The listing builds one solid part. Answer for the finished solid, in the listing's coordinates (mm). A direction names the side the tool comes from. Give positions to 0.01 mm unless a question says otherwise; leave off trailing zeros. Write each loop counter-clockwise with the first axis right and the second up, starting at its lowest first coordinate (ties: lowest second). Pieces come first, ordered by that corner, then holes.
```python
from build123d import *

# Parameters (mm, degrees)
BOSS_EXTRUDE1_DEPTH = 1.524


with BuildPart() as part:
    # Sketch1 → Boss-Extrude1 (new body)
    with BuildSketch(Plane.XY):
        with BuildLine():
            Line((82.44470135, -1.524), (82.44470135, 0))
            Line((82.44470135, 0), (51.403450054, 0))
            ThreePointArc((51.403450054, 0), (63.788927887, 14.019916875), (82.44470135, 12.634187153))
            ThreePointArc((82.44470135, 12.634187153), (98.093428139, 9.137765846), (111.269499156, 0))
            Line((111.269499156, 0), (111.269499156, -1.524))
            ThreePointArc((111.269499156, -1.524), (98.093428139, -10.661765846), (82.44470135, -14.158187153))
            ThreePointArc((82.44470135, -14.158187153), (63.788927887, -15.543916875), (51.403450054, -1.524))
            Line((51.403450054, -1.524), (82.44470135, -1.524))
        make_face()
    extrude(amount=BOSS_EXTRUDE1_DEPTH)


solid = part.part
```
Item 1: A cutting plane is placed at A-A, the plane x = 68. Give the vertices of the cut face in (y, z).
Conclusion:
outline: (-16.76, 0) - (-1.52, 0) - (-1.52, 1.52) - (-16.76, 1.52) - close; (0, 0) - (15.24, 0) - (15.24, 1.52) - (0, 1.52) - close
Item 2: Determine the mould class of faces 3 (the face through (97.886, 9.228, 0.751)), 4 (the face through (82, -4, 1.524)), 5 (the face through (67, -1.524, 1)) for opening direction Y: pulls with the +Y half, pulls with the -Y half, needs draft (parallel to the pull), parting line crosses it, or undercut.
Conclusion:
face 3: pulls with the +Y half
face 4: needs draft
face 5: undercut
Item 3: A cutting plane is placed at C-C, the plane x = 61.5. Give the vertices of the cut face in (y, z), plus the area to 3 significant figures.
Conclusion:
outline: (-14.45, 0) - (-1.52, 0) - (-1.52, 1.52) - (-14.45, 1.52) - close; (0, 0) - (12.92, 0) - (12.92, 1.52) - (0, 1.52) - close
area: 39.4 mm2
Item 4: Consider probe 1 along Y at (x, z) = (80, 1.25); probe 2 along Y at (x, z) = (73, 0.55); probe 3 along X at (y, z) = (2, 0.9). Determine where each line is inside the solid, lowest interval first.
Conclusion:
probe 1: y = -15.4 to -1.52, 0 to 13.87
probe 2: y = -17.06 to -1.52, 0 to 15.53
probe 3: x = 52.05 to 109.19
Item 5: A cutting plane is placed at B-B, the plane z = 1.05. Give the vertices of the cut face in (x, y), plus the area to 3 significant figures.
Conclusion:
outline: (51.4, -1.52) arc R21.04 ccw to (82.44, -14.16) arc R41.74 ccw to (111.27, -1.52) - (111.27, 0) arc R41.74 ccw to (82.44, 12.63) arc R21.04 ccw to (51.4, 0) - (82.44, 0) - (82.44, -1.52) - close
area: 1,320 mm2
Item 6: Which of the six approach directions +Z, -Z, +X, -X, +Y, -Y give full straight-line access (tool end or side, diameter ignored) to faces 1 (the face through (82, -4, 0)), 2 (the face through (67, 0, 1))?
Conclusion:
face 1: -Z, +X, -X, +Y, -Y
face 2: +Z, -Z, -X
Item 7: Each of these flat-tipped pins is pushed along its axis until it touches: P1, Ø0.8, axis at x = 67.5, z = 1, coming from the +Y side; P2, Ø0.5, axis at x = 61, z = 0.5, coming from the -Y side; P3, Ø0.8, axis at y = -0.5, z = 0.5, coming from the -X side. Where does it stop, or does it pass through?
Conclusion:
P1: stops at y = 15.22
P2: stops at y = -14.31
P3: stops at x = 82.44
Item 8: A cutting plane is placed at D-D, the plane y = -8. Give the vertices of the cut face in (x, z).
Conclusion:
outline: (54.4, 0) - (103.18, 0) - (103.18, 1.52) - (54.4, 1.52) - close
